```python
from build123d import *

# Parameters (mm, degrees)
SKETCH_1_W          = 70
SKETCH_1_H          = 50
EXTRUDE_1_DEPTH     = 6
SKETCH_2_W          = 2
SKETCH_2_H          = 50
EXTRUDE_2_DEPTH     = 24.5
SKETCH_3_R          = 2.25
CUT_EXTRUDE_1_DEPTH = 53.440442409


with BuildPart() as part:
    # 草图1 → 凸台-拉伸1 (new body)
    with BuildSketch(Plane(origin=(0, 0, 0), x_dir=(1, 0, 0), z_dir=(0, 1, 0))):
        Rectangle(SKETCH_1_W, SKETCH_1_H)
    extrude(amount=EXTRUDE_1_DEPTH)

    # 草图2 → 凸台-拉伸2 (add)
    with BuildSketch(Plane(origin=(0, 5.5, 0), x_dir=(1, 0, 0), z_dir=(0, 1, 0))):
        with Locations((-24, 0)):
            Rectangle(SKETCH_2_W, SKETCH_2_H)
        with Locations((-16, 0)):
            Rectangle(SKETCH_2_W, SKETCH_2_H)
        with Locations((-8, 0)):
            Rectangle(SKETCH_2_W, SKETCH_2_H)
        Rectangle(SKETCH_2_W, SKETCH_2_H)
        with Locations((8, 0)):
            Rectangle(SKETCH_2_W, SKETCH_2_H)
        with Locations((16, 0)):
            Rectangle(SKETCH_2_W, SKETCH_2_H)
        with Locations((24, 0)):
            Rectangle(SKETCH_2_W, SKETCH_2_H)
    extrude(amount=EXTRUDE_2_DEPTH)

    # 草图3 → 切除-拉伸1 (cut, through all)
    with BuildSketch(Plane(origin=(0, 30, 0), x_dir=(1, 0, 0), z_dir=(0, 1, 0))):
        with Locations(Location((-31.5, 15, 0), (0, 0, 270))):
            Circle(SKETCH_3_R)
        with Locations(Location((-31.5, -15, 0), (0, 0, 270))):
            Circle(SKETCH_3_R)
        with Locations(Location((31.5, 15, 0), (0, 0, 270))):
            Circle(SKETCH_3_R)
        with Locations(Location((31.5, -15, 0), (0, 0, 270))):
            Circle(SKETCH_3_R)
    extrude(amount=-CUT_EXTRUDE_1_DEPTH, mode=Mode.SUBTRACT)


solid = part.part
```
Part model, mm, in its own coordinate system. A direction names the side the tool comes from. Give positions to 0.01 mm unless a question says otherwise; leave off trailing zeros. Order: outer loops, then holes, each group sorted by start corner. A loop starts at its lowest first (then second) coordinate and runs counter-clockwise, first axis right, second up. Notation, with made-up numbers: (-12, 28.5) - (20, 28.5) arc R8 cw to (20, 38.5) - close; hole circle Ø6 at (7.5, -1.5). An arc over 180 degrees is marked (long way). Use one line per item in the form item = value.
Item 1: Probe probe 1 along X at (y, z) = (2.05, -15); probe 2 along Y at (x, z) = (-30.5, 11.5). List the from-to ranges inside material, lowest first. Write a range as from..to.
Solution:
probe_1 = -35..-33.75, -29.25..29.25, 33.75..35
probe_2 = 0..6
Item 2: Slice it at A-A on y = 18.25. Give the cut face in (x, z).
Solution:
outline = (-25, -25) - (-23, -25) - (-23, 25) - (-25, 25) - close; (-17, -25) - (-15, -25) - (-15, 25) - (-17, 25) - close; (-9, -25) - (-7, -25) - (-7, 25) - (-9, 25) - close; (-1, -25) - (1, -25) - (1, 25) - (-1, 25) - close; (7, -25) - (9, -25) - (9, 25) - (7, 25) - close; (15, -25) - (17, -25) - (17, 25) - (15, 25) - close; (23, -25) - (25, -25) - (25, 25) - (23, 25) - close
Item 3: Which spindle directions (+Z, -Z, +X, -X, +Y, -Y) get a long thin tool onto all of the face, cutting with end or side? Do faces 5 (the face through (8, 30, 0)), 6 (the face through (9, 18, 0)). Say none if no direction does.
Solution:
face_5 = +Z, -Z, +X, -X, +Y
face_6 = +Z, -Z, +Y
Item 4: Pin check, flat tips, straight feed: pin 1 Ø3.5 at (x, z) = (-31.5, 15) entering from +Y; pin 2 Ø7 at (y, z) = (18, 6) entering from +X; pin 3 Ø3 at (x, z) = (13, -2.5) entering from +Y; pin 4 Ø4 at (y, z) = (22.5, 19) entering from -X. Stop position of each tip, or through.
Solution:
pin_1 = through
pin_2 = 25
pin_3 = 6
pin_4 = -25
Item 5: Two-plate mould, pull along Z, no slides. Class faces 1 (the face through (0, 15, 25)), 2 (the face through (-16, 30, 0)), 3 (the face through (33.397, 3.042, 16.21)), 4 (the face through (-30.824, 3.042, -12.854)): released by +Z, released by -Z, zero draft, split by the parting line, or undercut.
Solution:
face_1 = released by +Z
face_2 = zero draft
face_3 = undercut
face_4 = undercut
Item 6: Slice it at D-D on z = 15. Count the separate pieces of the cut face and the enclosed holes in it, and give its area (3 significant figures).
Solution:
separate_pieces = 3
enclosed_holes = 0
area = 702 mm2
Item 7: Slice it at B-B on x = -31.5. Give the cut face in (y, z), and give its area (3 significant figures).
Solution:
outline = (0, -25) - (6, -25) - (6, -17.25) - (0, -17.25) - close; (0, -12.75) - (6, -12.75) - (6, 12.75) - (0, 12.75) - close; (0, 17.25) - (6, 17.25) - (6, 25) - (0, 25) - close
area = 246 mm2
